For this review, take the finished solid that the model builds, in its own axes (mm). Face numbers are marked on the shaded views. Give positions to 0.01 mm unless a question says otherwise; leave off trailing zeros. Order: outer loops, then holes, each group sorted by start corner. A loop starts at its lowest first (then second) coordinate and runs counter-clockwise, first axis right, second up. Notation, with made-up numbers: (20, 11.5) -> (65, 11.5) arc R33 cw to (65, 40.5) -> close; hole circle Ø10 at (49, 9). An arc over 180 degrees is marked (long way). One line per item, written item: value. Start each with the question number.
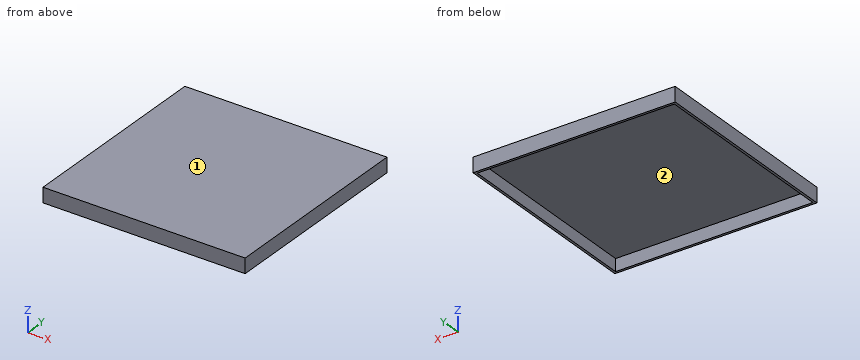
from build123d import *

# Parameters (mm, degrees)
SKETCH_2_W      = 164
SKETCH_2_H      = 164
EXTRUDE_1_DEPTH = 12
SKETCH_1_W      = 160
SKETCH_1_H      = 160
EXTRUDE_2_DEPTH = 10


with BuildPart() as part:
    # 草图2 → 凸台-拉伸1 (new body)
    with BuildSketch(Plane.XY):
        with Locations((-72.7457284, 11.344743276)):
            Rectangle(SKETCH_2_W, SKETCH_2_H)
    extrude(amount=EXTRUDE_1_DEPTH)


with BuildPart() as body_2:
    # 草图1 → 凸台-拉伸2 (new body)
    with BuildSketch(Plane.XY):
        with Locations((-72.7457284, 11.344743276)):
            Rectangle(SKETCH_1_W, SKETCH_1_H)
    extrude(amount=EXTRUDE_2_DEPTH)


with BuildPart() as part_1:
    add(part.part)

    # Combine 1: cut body 2
    add(body_2.part, mode=Mode.SUBTRACT)


solid = part_1.part
Q1. Take a section at B-B (y = -20). State the section outline as (x, z) points.
Q2. Take a section at C-C (x = -18.5). State the section outline as (y, z) points.
Q3. For line 1 along Y through (x, z) = (-62, 9.25); line 2 along X through (y, z) = (56.5, 7.5); line 3 along Z through (x, y) = (-107.5, 82), list the stretches that pass through material, from the lowest coordinate up.
Q4. For pin 1 Ø5 at (x, y) = (-25, -45) entering from -Z, flat-tipped, find the tip position at first contact; note if it passes through.
Q5. Take a section at A-A (z = 6). State the section outline as (x, y) points.
Q6. Mouldability with a two-part tool opening along Y and no side actions: class the marked faces 1 and 2 as pulls with the +Y half, pulls with the -Y half, needs draft (parallel to the pull), parting line crosses it, or undercut.
Answers below:
1. outline: (-154.75, 0) -> (-152.75, 0) -> (-152.75, 10) -> (7.25, 10) -> (7.25, 0) -> (9.25, 0) -> (9.25, 12) -> (-154.75, 12) -> close
2. outline: (-70.66, 0) -> (-68.66, 0) -> (-68.66, 10) -> (91.34, 10) -> (91.34, 0) -> (93.34, 0) -> (93.34, 12) -> (-70.66, 12) -> close
3. line 1: y = -70.66 to -68.66, 91.34 to 93.34
3. line 2: x = -154.75 to -152.75, 7.25 to 9.25
3. line 3: z = 10 to 12
4. pin 1: stops at z = 10
5. outline: (-154.75, -70.66) -> (9.25, -70.66) -> (9.25, 93.34) -> (-154.75, 93.34) -> close; hole (-152.75, -68.66) -> (7.25, -68.66) -> (7.25, 91.34) -> (-152.75, 91.34) -> close
6. face 1: needs draft
6. face 2: undercut
